```python
from build123d import *

# Parameters (mm, degrees)
SKETCH_1_R                       = 8
EXTRUDE_1_DEPTH                  = 1.6
SKETCH_2_R                       = 7.165
EXTRUDE_2_DEPTH                  = 10
CUT_EXTRUDE_1_DEPTH              = 12.6
CUT_EXTRUDE_2_DEPTH              = 10
FILLET_1_R                       = 0.305
PATTERN_CIRCULAR_1_COUNT         = 9
FILLET_1_OF_PATTERN_CIRCULAR_1_R = 0.305


with BuildPart() as part:
    # Sketch 1 → Extrude 1 (new body)
    with BuildSketch(Plane(origin=(0, 0, 0), x_dir=(1, 0, 0), z_dir=(0, 1, 0))):
        Circle(SKETCH_1_R)
    extrude(amount=EXTRUDE_1_DEPTH)

    # Sketch 2 → Extrude 2 (add)
    with BuildSketch(Plane(origin=(0, 1.6, 0), x_dir=(1, 0, 0), z_dir=(0, 1, 0))):
        Circle(SKETCH_2_R)
    extrude(amount=EXTRUDE_2_DEPTH)

    # Sketch 3 → Cut-Extrude 1 (cut, through all)
    with BuildSketch(Plane(origin=(0, 11.6, 0), x_dir=(1, 0, 0), z_dir=(0, 1, 0))):
        with BuildLine():
            Line((1.987460691, 3.7), (-1.987460691, 3.7))
            ThreePointArc((-1.987460691, 3.7), (-2.155535327, -3.604673002), (4.2, 0))
            ThreePointArc((4.2, 0), (3.604673002, 2.155535327), (1.987460691, 3.7))
        make_face()
    extrude(amount=-CUT_EXTRUDE_1_DEPTH, mode=Mode.SUBTRACT)

    # Sketch 4 → Cut-Extrude 2 (cut)
    with BuildSketch(Plane(origin=(0, 11.6, 0), x_dir=(1, 0, 0), z_dir=(0, 1, 0))):
        with BuildLine():
            Line((-1.702574257, 6.959774845), (-1.51531734, 6.19430692))
            ThreePointArc((-1.51531734, 6.19430692), (2.8e-08, 5.005), (1.515317353, 6.194306973))
            Line((1.515317353, 6.194306973), (1.702574257, 6.959774845))
            ThreePointArc((1.702574257, 6.959774845), (0, 7.165), (-1.702574257, 6.959774845))
        make_face()
    cut_extrude_2 = extrude(amount=-CUT_EXTRUDE_2_DEPTH, mode=Mode.SUBTRACT)

    # Fillet 1
    fillet_1_edges = [part.edges().sort_by_distance(p)[0] for p in [
        (-1.702574257, 6.6, -6.959774845),
        (1.702574257, 6.6, -6.959774845),
    ]]
    fillet(fillet_1_edges, radius=FILLET_1_R)

    # Pattern Circular 1: Cut-Extrude 2 ×9 about axis
    pattern_circular_1_axis = Axis((0, 0, 0), (0, 1, 0))
    for i in range(1, PATTERN_CIRCULAR_1_COUNT):
        add(cut_extrude_2.rotate(pattern_circular_1_axis, i * 360 / PATTERN_CIRCULAR_1_COUNT), mode=Mode.SUBTRACT)

    # Fillet 1 of Pattern Circular 1
    fillet_1_of_pattern_circular_1_edges = [part.edges().sort_by_distance(p)[0] for p in [
        (-5.777904586, 6.6, -4.237103208),
        (-3.169409488, 6.6, -6.425890483),
        (-7.149689144, 6.6, 0.46815611),
        (-6.55839131, 6.6, -2.885260548),
        (-5.176054692, 6.6, 4.954359981),
        (-6.878628949, 6.6, 2.005414864),
        (-0.780486724, 6.6, 7.122363756),
        (-3.980279656, 6.6, 5.957734373),
        (3.980279656, 6.6, 5.957734373),
        (0.780486724, 6.6, 7.122363756),
        (6.878628949, 6.6, 2.005414864),
        (5.176054692, 6.6, 4.954359981),
        (6.55839131, 6.6, -2.885260548),
        (7.149689144, 6.6, 0.46815611),
        (3.169409488, 6.6, -6.425890483),
        (5.777904586, 6.6, -4.237103208),
    ]]
    fillet(fillet_1_of_pattern_circular_1_edges, radius=FILLET_1_OF_PATTERN_CIRCULAR_1_R)


solid = part.part
```
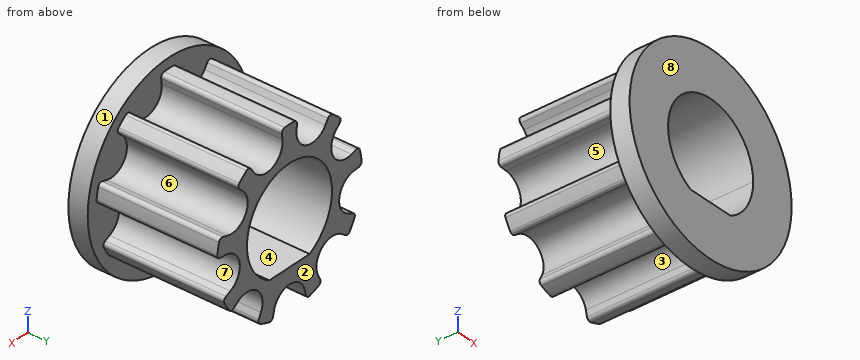
The listing builds one solid part. Answer for the finished solid, in the listing's coordinates (mm). Face numbers are marked on the shaded views. A direction names the side the tool comes from. Coordinates: 2 decimals unless noted, no trailing zeros. Loops run counter-clockwise (first coordinate to the right, second up) from the corner with the lowest first, then second, coordinate; pieces in that order, holes last. Notation, with made-up numbers: (-39, 15.5) -> (9, 15.5) arc R25 ccw to (9, 53.5) -> close; hole circle Ø3 at (-18.5, 52). An arc over 180 degrees is marked (long way). Return JSON: item names as keys, results as strings. Group by question number.
(1) A cutting plane is placed at A-A on z = 2.5. Write down the section's boundary in (x, y).
(2) Which of the six approach directions +Z, -Z, +X, -X, +Y, -Y give full straight-line access (tool end or side, diameter ignored) to the marked faces 5, 6, 7 and 8?
(3) A cutting plane is placed at B-B on x = 0. Write down the section's boundary in (y, z) (3 decimals), and give its area (3 significant figures).
(4) Given pin 1 Ø2 at (x, y) = (0.5, 7) entering from +Z (3 decimals); pin 2 Ø1 at (y, z) = (1.5, -1) entering from +X; pin 3 Ø5 at (y, z) = (9, 1.5) entering from -X, each flat-ended and moving along its own axis, determine where each tip first touches the part or whether it passes through.
(5) Determine the mould class of the marked faces 1, 2, 3 and 4 for opening direction Z: released by +Z, released by -Z, zero draft, split by the parting line, or undercut.
(6) A cutting plane is placed at C-C on z = -5.5. Write down the section's boundary in (x, y), and give its area (3 significant figures).
(7) Find the intervals of material crossed by probe 1 along X at (y, z) = (3.25, 4.75); probe 2 along Z at (x, y) = (0, 9.25) (3 decimals); probe 3 along Y at (x, z) = (-7, 3), in increasing order. Write a range as from..to.
The answers:
{
 "1": {"outline": "(-7.6, 0) -> (-3.37, 0) -> (-3.37, 11.6) -> (-4.34, 11.6) -> (-4.34, 1.6) -> (-7.6, 1.6) -> close; (3.37, 0) -> (7.6, 0) -> (7.6, 1.6) -> (4.34, 1.6) -> (4.34, 11.6) -> (3.37, 11.6) -> close"},
 "2": {"face 5": "-X, +Y", "face 6": "+Y", "face 7": "+X, +Y", "face 8": "+Z, -Z, +X, -X, -Y"},
 "3": {"outline": "(0, -8) -> (1.6, -8) -> (1.6, -5.005) -> (11.6, -5.005) -> (11.6, -3.7) -> (0, -3.7) -> close; (0, 4.2) -> (11.6, 4.2) -> (11.6, 7.165) -> (1.6, 7.165) -> (1.6, 8) -> (0, 8) -> close", "area": "55.7 mm^2"},
 "4": {"pin 1": "stops at z = 7.165", "pin 2": "stops at x = 7.98", "pin 3": "stops at x = -7.12"},
 "5": {"face 1": "split by the parting line", "face 2": "zero draft", "face 3": "released by -Z", "face 4": "undercut"},
 "6": {"outline": "(-5.81, 0) -> (5.81, 0) -> (5.81, 1.6) -> (2.73, 1.6) -> (2.73, 11.6) -> (1.14, 11.6) -> (1.14, 1.6) -> (-1.14, 1.6) -> (-1.14, 11.6) -> (-2.73, 11.6) -> (-2.73, 1.6) -> (-5.81, 1.6) -> close", "area": "50.4 mm^2"},
 "7": {"probe 1": "x = -4.96..-2.89, -1.6..1.6, 2.89..4.96", "probe 2": "z = -5.005..-3.7, 4.2..7.165", "probe 3": "y = 0..1.6"}
}
